The model under review builds one solid part; all positions refer to its coordinate system, in mm. Coordinates: 2 decimals unless noted, no trailing zeros. Write each loop counter-clockwise with the first axis right and the second up, starting at its lowest first coordinate (ties: lowest second). Pieces come first, ordered by that corner, then holes. Notation, with made-up numbers: (56.25, 51.5) - (62.25, 51.5) arc R10 ccw to (62.25, 68.5) - close; hole circle Ø3 at (-37, 33.5). An arc over 180 degrees is marked (long way). Return JSON: item names as keys, results as strings. Group by question number.
(1) We need section C-C on x = 6. State the section outline as (y, z) points.
(2) We need section A-A on z = 32.5. State the section outline as (x, y) points, then the cut area to 3 significant figures.
(3) We need section B-B on x = 47.5. State the section outline as (y, z) points.
(4) For pin 1 Ø14.5 at (x, z) = (27.5, 32.5) entering from +Y; pin 2 Ø1.5 at (y, z) = (2, 62) entering from -X; pin 3 Ø3 at (x, y) = (10.5, 1.5) entering from -Z; pin 4 Ø1.5 at (x, y) = (29.5, 3.5) entering from +Z, all flat-tipped, find the tip position at first contact; note any pin that passes through.
(5) We need section D-D on y = 1.95. Give the number of separate pieces and of enclosed holes in the cut face, then the cut area to 3 significant figures.
(6) To check wall thickness, follow L1, parallel to Z at x = 5, y = 2.15; L2, parallel to Z at x = 10, y = 4.15; L3, parallel to X at y = 2, z = 52.5. State the ranges of each line that lie inside material, in increasing order. Write a range as from..to.
```python
from build123d import *

# Parameters (mm, degrees)
BOSS_EXTRU_1_DEPTH      = 5
ESQUISSE2_R             = 8
ENL_V_MAT_EXTRU_1_DEPTH = 10
ENL_V_MAT_EXTRU_2_DEPTH = 10
ESQUISSE4_R             = 3
ENL_V_MAT_EXTRU_3_DEPTH = 10


with BuildPart() as part:
    # Esquisse1 → Boss.-Extru.1 (new body)
    with BuildSketch(Plane(origin=(0, 0, 0), x_dir=(1, 0, 0), z_dir=(0, 1, 0))):
        Polygon((17.5, -5), (37.5, -5), (37.5, 0), (55, 0), (55, -60), (55, -65), (37.5, -65), (37.5, -60), (17.5, -60), (17.5, -65), (0, -65), (0, -60), (0, -42.5), (-5, -42.5), (-5, -22.5), (0, -22.5), (0, 0), (17.5, 0), align=None)
    extrude(amount=BOSS_EXTRU_1_DEPTH)

    # Esquisse2 → Enlèv. mat.-Extru.1 (cut)
    with BuildSketch(Plane(origin=(0, 5, 0), x_dir=(1, 0, 0), z_dir=(0, 1, 0))):
        with Locations((27.5, -32.5)):
            Circle(ESQUISSE2_R)
    extrude(amount=-ENL_V_MAT_EXTRU_1_DEPTH, mode=Mode.SUBTRACT)

    # Esquisse3 → Enlèv. mat.-Extru.2 (cut)
    with BuildSketch(Plane(origin=(0, 5, 0), x_dir=(1, 0, 0), z_dir=(0, 1, 0))):
        Polygon((13, -5.9), (11, -5.9), (11, -4.75), (8.5, -4.75), (8.5, -5.9), (0, -5.9), (0, -9.1), (8.5, -9.1), (8.5, -10.25), (11, -10.25), (11, -9.1), (13, -9.1), align=None)
    enl_v_mat_extru_2 = extrude(amount=-ENL_V_MAT_EXTRU_2_DEPTH, mode=Mode.SUBTRACT)

    # Symétrie1: Enlèv. mat.-Extru.2 across plane
    add(enl_v_mat_extru_2.mirror(Plane(origin=(0, 0, 32.5), x_dir=(1, 0, 0), z_dir=(0, 0, -1))), mode=Mode.SUBTRACT)

    # Esquisse4 → Enlèv. mat.-Extru.3 (cut)
    with BuildSketch(Plane(origin=(0, 5, 0), x_dir=(1, 0, 0), z_dir=(0, 1, 0))):
        with Locations((47.5, -52.5)):
            Circle(ESQUISSE4_R)
    extrude(amount=-ENL_V_MAT_EXTRU_3_DEPTH, mode=Mode.SUBTRACT)


solid = part.part
```
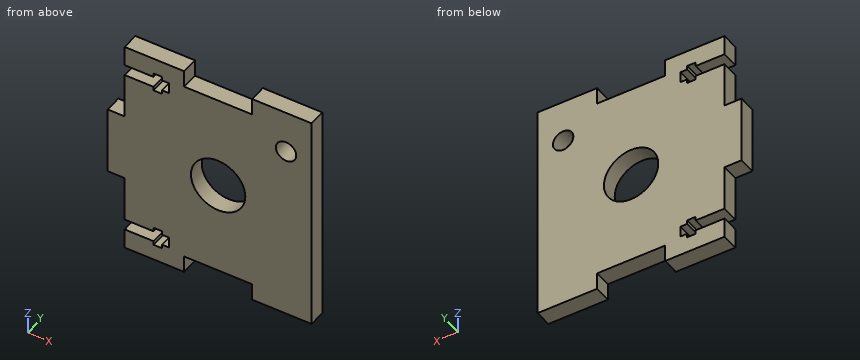
Ans:
{
 "1": {"outline": "(0, 0) - (5, 0) - (5, 5.9) - (0, 5.9) - close; (0, 9.1) - (5, 9.1) - (5, 55.9) - (0, 55.9) - close; (0, 59.1) - (5, 59.1) - (5, 65) - (0, 65) - close"},
 "2": {"outline": "(-5, 0) - (19.5, 0) - (19.5, 5) - (-5, 5) - close; (35.5, 0) - (55, 0) - (55, 5) - (35.5, 5) - close", "area": "220 mm²"},
 "3": {"outline": "(0, 0) - (5, 0) - (5, 49.5) - (0, 49.5) - close; (0, 55.5) - (5, 55.5) - (5, 65) - (0, 65) - close"},
 "4": {"pin 1": "through", "pin 2": "x = 0", "pin 3": "z = 0", "pin 4": "z = 60"},
 "5": {"separate pieces": "1", "enclosed holes": "2", "area": "3,150 mm²"},
 "6": {"L1": "0..5.9, 9.1..55.9, 59.1..65", "L2": "0..4.75, 10.25..54.75, 60.25..65", "L3": "0..44.5, 50.5..55"}
}
